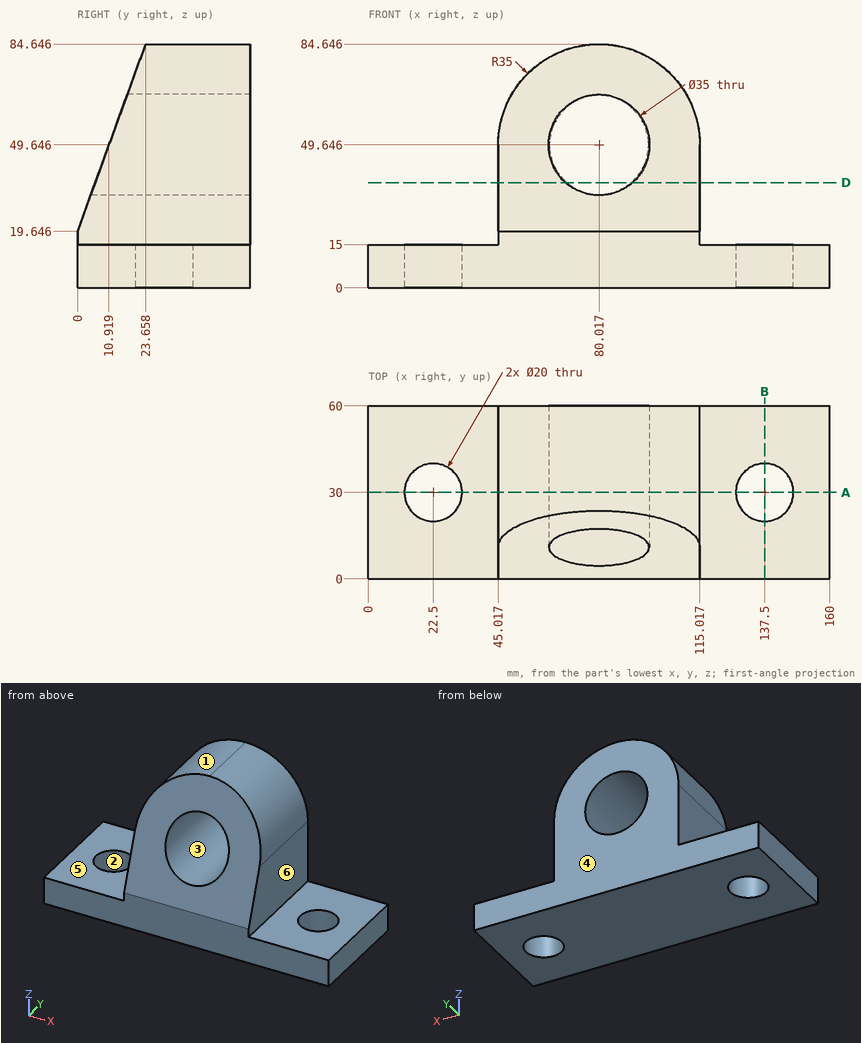
Can you work these out from the drawing? Everything is in mm from the part's minimum corner. A direction names the side the tool comes from. Round coordinates to 2 decimals unless told otherwise and drop trailing zeros. Write each loop counter-clockwise with the first axis right and the second up, starting at its lowest first coordinate (ties: lowest second). Pieces come first, ordered by that corner, then holes. Notation, with made-up numbers: M 41,50 L 61,50 A10 ccw 61,54 Z; hole C 0.5,65 d1. An arc over 180 degrees is marked long. Use a Markdown table: item, result.
Item 1: If I drill on line 1 along Y through (x, z) = (137, 10); line 2 along Z through (x, y) = (144, 50.5); line 3 along X through (y, z) = (52.5, 20.5), over which ranges is the centre line in solid material (lowest first)? Write a range as [from, to].
Found:
| item | result |
|---|---|
| line 1 | y = [0, 20.01], [39.99, 60] |
| line 2 | z = [0, 15] |
| line 3 | x = [45.02, 115.02] |
Item 2: I want a section at A-A (y = 30). State how many separate pieces and enclosed holes the cut face has, and give its area (3 significant figures).
Found:
| item | result |
|---|---|
| separate pieces | 3 |
| enclosed holes | 1 |
| area | 5,190 mm2 |
Item 3: We'd pull the mould along Z, two halves only. Please class the marked faces 1, 2 and 3: released by +Z, released by -Z, zero draft, split by the parting line, or undercut.
Found:
| item | result |
|---|---|
| face 1 | released by +Z |
| face 2 | zero draft |
| face 3 | undercut |
Item 4: Which directions (+Z, -Z, +X, -X, +Y, -Y) give clear straight access to the entire face, cutting with the end or side of a thin tool? Please do the marked faces 4, 5 and 6.
Found:
| item | result |
|---|---|
| face 4 | +Z, -Z, +X, -X, +Y |
| face 5 | +Z, -X, +Y, -Y |
| face 6 | +Z, +X, +Y, -Y |
Item 5: I want a section at B-B (x = 137.5). List the corners of the cut face in (y, z) for me.
Found:
| item | result |
|---|---|
| outline | M 0,0 L 20,0 L 20,15 L 0,15 Z; M 40,0 L 60,0 L 60,15 L 40,15 Z |
Item 6: I want a section at D-D (z = 36.5). List the corners of the cut face in (x, y) for me (1 decimal).
Found:
| item | result |
|---|---|
| outline | M 45,6.1 L 68.5,6.1 L 68.5,60 L 45,60 Z; M 91.6,6.1 L 115,6.1 L 115,60 L 91.6,60 Z |
Item 7: For pin 1 Ø21 at (x, z) = (80.02, 49.65) entering from +Y; pin 2 Ø2 at (x, y) = (100.5, 40) entering from -Z; pin 3 Ø1 at (y, z) = (49, 72.5) entering from -X (1 decimal); pin 4 Ø1.5 at (y, z) = (20.5, 52) entering from +X, each with a flat end and sliding along its axis, tell me the tip position at first contact or that it passes through.
Found:
| item | result |
|---|---|
| pin 1 | passes through |
| pin 2 | stops at z = 0 |
| pin 3 | stops at x = 53.1 |
| pin 4 | stops at x = 114.98 |
